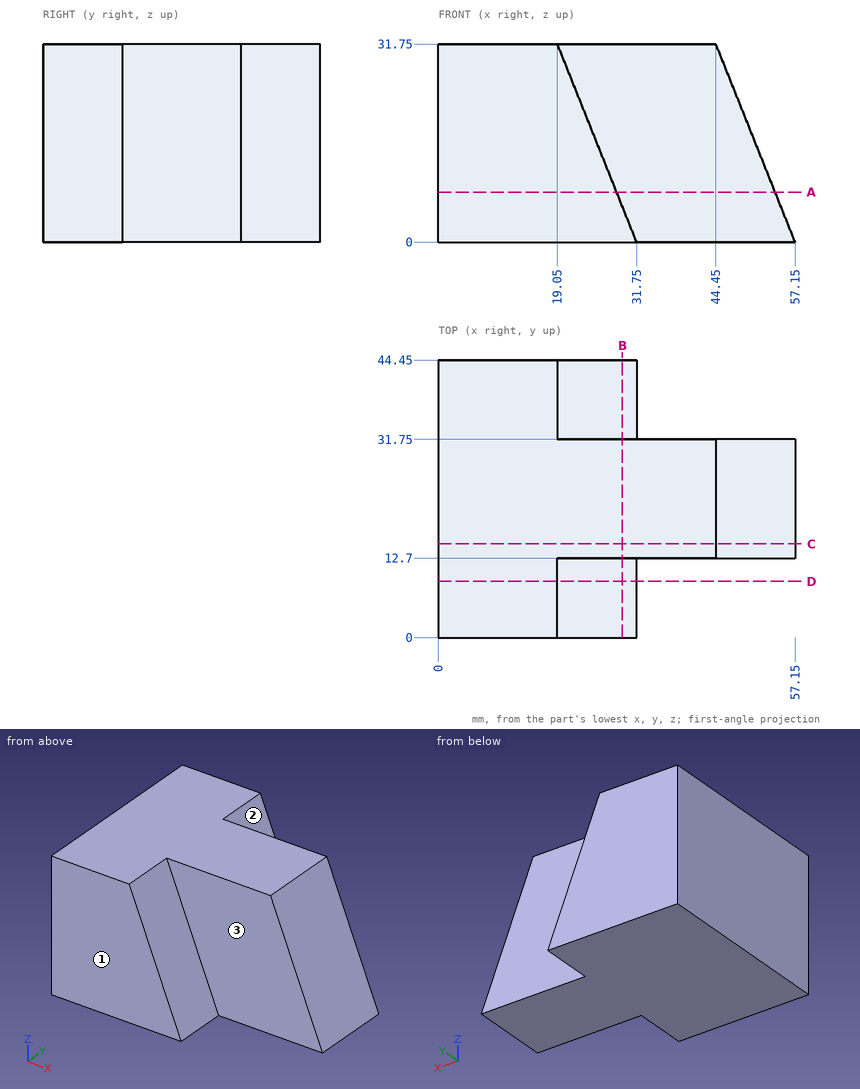
For this review, use the dimensioned drawing (mm, ordinates from the lowest corner) and the shaded views. A direction names the side the tool comes from. Round coordinates to 2 decimals unless told otherwise and drop trailing zeros. Write each loop counter-clockwise with the first axis right and the second up, starting at its lowest first coordinate (ties: lowest second). Pieces come first, ordered by that corner, then holes. Notation, with made-up numbers: (5, -23.5) -> (26, -23.5) arc R18 ccw to (26, 5.5) -> close; hole circle Ø6 at (59.25, 81.25). An arc over 180 degrees is marked (long way). One line per item, written item: value. Start each with the question number.
Q1. Insertion check: P1, Ø12, axis at y = 39.5, z = 25.5, coming from the +X side; P2, Ø6, axis at x = 41.5, z = 10.5, coming from the +Y side; P3, Ø3, axis at y = 26, z = 4.5, coming from the +X side. Each pin has a flat end and moves straight along its axis. Give the tip position at first contact, or say it passes through.
Q2. Add section B-B (x = 29.5). Give the boundary of the cut face in (y, z) (3 decimals), then the cut area to 3 significant figures.
Q3. Add section D-D (y = 9). Give the boundary of the cut face in (x, z).
Q4. Tool access review of the marked faces 1, 2 and 3: name each direction out of +Z, -Z, +X, -X, +Y, -Y from which nothing blocks a thin tool from reaching the whole face with its end or side.
Q5. Add section A-A (z = 8). Give the boundary of the cut face in (x, y).
Q6. To check wall thickness, follow probe 1 along Y at (x, z) = (36, 6); probe 2 along X at (y, z) = (6, 3.5); probe 3 along X at (y, z) = (12.5, 23). State the ranges of each line that lie inside material, in increasing order.
Q7. Add section C-C (y = 15). Give the boundary of the cut face in (x, z).
Response:
1. P1: stops at x = 23.95
1. P2: stops at y = 31.75
1. P3: stops at x = 55.95
2. outline: (0, 0) -> (44.45, 0) -> (44.45, 5.625) -> (31.75, 5.625) -> (31.75, 31.75) -> (12.7, 31.75) -> (12.7, 5.625) -> (0, 5.625) -> close
2. area: 748 mm^2
3. outline: (0, 0) -> (31.75, 0) -> (19.05, 31.75) -> (0, 31.75) -> close
4. face 1: +Z, -Z, +X, -X, -Y
4. face 2: +Z, +X, +Y
4. face 3: +Z, +X, -Y
5. outline: (0, 0) -> (28.55, 0) -> (28.55, 12.7) -> (53.95, 12.7) -> (53.95, 31.75) -> (28.55, 31.75) -> (28.55, 44.45) -> (0, 44.45) -> close
6. probe 1: y = 12.7 to 31.75
6. probe 2: x = 0 to 30.35
6. probe 3: x = 0 to 22.55
7. outline: (0, 0) -> (57.15, 0) -> (44.45, 31.75) -> (0, 31.75) -> close
